from build123d import *

# Parameters (mm, degrees)
SKETCH_R      = 7
PAD_DEPTH     = 16
SKETCH001_R   = 7
SKETCH001_R_2 = 2.5
PAD001_DEPTH  = 13


with BuildPart() as part:
    # Sketch → Pad (new body)
    with BuildSketch(Plane.XY):
        Circle(SKETCH_R)
        Polygon((4.330127, 0), (2.165064, 3.75), (-2.165064, 3.75), (-4.330127, 0), (-2.165064, -3.75), (2.165064, -3.75), align=None, mode=Mode.SUBTRACT)
    extrude(amount=PAD_DEPTH)

    # Sketch001 → Pad001 (join)
    with BuildSketch(Plane.XY):
        Circle(SKETCH001_R)
        Circle(SKETCH001_R_2, mode=Mode.SUBTRACT)
    extrude(amount=PAD001_DEPTH)


solid = part.part
Verification items for the finished model (mm, model axes). A direction names the side the tool comes from. Coordinates: 2 decimals unless noted, no trailing zeros. Order: outer loops, then holes, each group sorted by start corner. A loop starts at its lowest first (then second) coordinate and runs counter-clockwise, first axis right, second up.
1. Go/stop test with flat-tipped pins: pin 1 Ø1 at (x, y) = (0.5, 2) entering from +Z; pin 2 Ø5 at (y, z) = (4.5, 5) entering from +X; pin 3 Ø4 at (x, z) = (-4, 12.5) entering from +Y. Record where each tip stops, or that it passes through.
Results found:
pin 1: stops at z = 13
pin 2: stops at x = 6.71
pin 3: stops at y = 6.71
2. Sectioned sample at C-C, the plane z = 3.5. Record the cut outline in (x, y), and give its area (3 significant figures).
Results found:
outline: circle Ø14 at (0, 0); hole circle Ø5 at (0, 0)
area: 134 mm2
3. Set-up check for faces 4 (the face through (-3.26, -1.85, 14.48)), 5 (the face through (0, -3, 0)): record each of +Z, -Z, +X, -X, +Y, -Y from which the full face is reachable in a straight line by a thin tool's end or side.
Results found:
face 4: +Z
face 5: -Z, +X, -X, +Y, -Y
4. Scan lines: line 1 (Y direction, x = 0, z = 3); line 2 (X direction, y = 3.25, z = 14.25); line 3 (Y direction, x = 5.5, z = 14.75). Record each from-to range of solid material in increasing order.
Results found:
line 1: y = -7 to -2.5, 2.5 to 7
line 2: x = -6.2 to -2.45, 2.45 to 6.2
line 3: y = -4.33 to 4.33
5. Sectioned sample at B-B, the plane y = 2. Record the cut outline in (x, z).
Results found:
outline: (-6.71, 0) - (-1.5, 0) - (-1.5, 13) - (-3.18, 13) - (-3.18, 16) - (-6.71, 16) - close; (1.5, 0) - (6.71, 0) - (6.71, 16) - (3.18, 16) - (3.18, 13) - (1.5, 13) - close
6. Sectioned sample at A-A, the plane x = 0. Record the cut outline in (y, z).
Results found:
outline: (-7, 0) - (-2.5, 0) - (-2.5, 13) - (-3.75, 13) - (-3.75, 16) - (-7, 16) - close; (2.5, 0) - (7, 0) - (7, 16) - (3.75, 16) - (3.75, 13) - (2.5, 13) - close
7. Sectioned sample at D-D, the plane y = -3.25. Record the cut outline in (x, z).
Results found:
outline: (-6.2, 0) - (6.2, 0) - (6.2, 16) - (2.45, 16) - (2.45, 13) - (-2.45, 13) - (-2.45, 16) - (-6.2, 16) - close
8. Release check for a two-part mould opening along Y. For faces 1 (the face through (3, -3, 16)), 2 (the face through (3.232, -1.901, 14.479)), 3 (the face through (6.466, -2.681, 7.888)) record: +Y half, -Y half, draft (parallel to the pull), parting line (faces both ways), or undercut.
Results found:
face 1: draft
face 2: undercut
face 3: parting line
